Could you check a few things on this drawing? It's one solid part, dimensions in mm from its lowest x, y, z. A direction names the side the tool comes from. Give positions to 0.01 mm unless a question says otherwise; leave off trailing zeros. Loops run counter-clockwise (first coordinate to the right, second up) from the corner with the lowest first, then second, coordinate; pieces in that order, holes last.
Q1. Suppose I cut it at C-C (x = 46). List the corners of the cut face in (y, z) for me, and give its area (3 significant figures).
Q2. I need wall thicknesses on probe 1 along Z at (x, y) = (46, 1.75); probe 2 along Y at (x, z) = (42, 8.25); probe 3 along X at (y, z) = (7.5, 0.5). Which ranges of each line are inside material? Lowest first, please.
Q3. Suppose I cut it at A-A (z = 5). List the corners of the cut face in (x, y) for me, and give its area (3 significant figures).
Q4. For the marked faces 4, 5 and 6, which set-ups out of +Z, -Z, +X, -X, +Y, -Y let a thin tool reach every point of the face, with its end or its side?
Q5. I'm going to push flat-ended pins straight in: P1, Ø6, axis at x = 11, z = 5.5, coming from the +Y side; P2, Ø6, axis at y = 8.5, z = 7.5, coming from the +X side; P3, Ø1.8, axis at y = 9, z = 4.5, coming from the +X side; P4, Ø3, axis at y = 9.5, z = 6.5, coming from the -X side. Where does each tip first touch, or does it pass through?
Q6. Thinking about a two-plate mould opening in X: for the marked faces 1, 2 and 3, which applies, pulls with the +X half, pulls with the -X half, needs draft (parallel to the pull), parting line crosses it, or undercut?
Q7. Suppose I cut it at D-D (z = 1.75). List the corners of the cut face in (x, y) for me.
Q8. Suppose I cut it at B-B (y = 4.25). List the corners of the cut face in (x, z) for me, and give its area (3 significant figures).
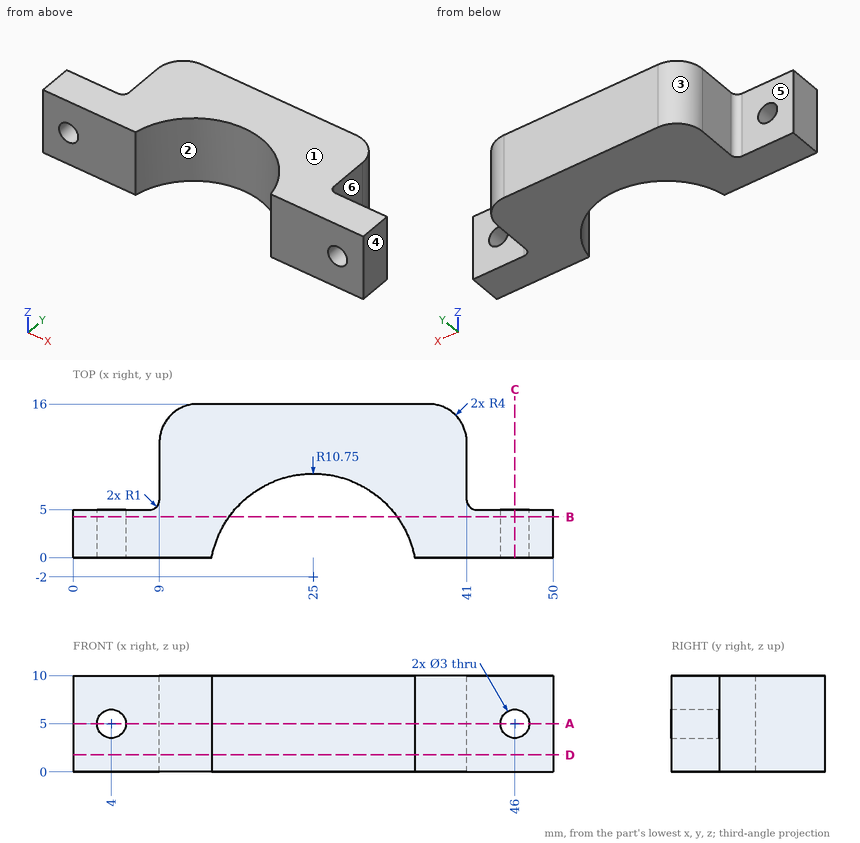
Solutions:
1. outline: (0, 0) - (5, 0) - (5, 3.5) - (0, 3.5) - close; (0, 6.5) - (5, 6.5) - (5, 10) - (0, 10) - close
1. area: 35.0 mm2
2. probe 1: z = 0 to 3.5, 6.5 to 10
2. probe 2: y = 0 to 5
2. probe 3: x = 9 to 19.97, 30.03 to 41
3. outline: (0, 0) - (2.5, 0) - (2.5, 5) - (0, 5) - close; (5.5, 0) - (14.44, 0) arc R10.75 cw to (35.56, 0) - (44.5, 0) - (44.5, 5) - (42, 5) arc R1 cw to (41, 6) - (41, 12) arc R4 ccw to (37, 16) - (13, 16) arc R4 ccw to (9, 12) - (9, 6) arc R1 cw to (8, 5) - (5.5, 5) - close; (47.5, 0) - (50, 0) - (50, 5) - (47.5, 5) - close
3. area: 427 mm2
4. face 4: +Z, -Z, +X, +Y, -Y
4. face 5: +Z, -Z, -X, +Y
4. face 6: +Z, -Z, +X, +Y
5. P1: stops at y = 16
5. P2: stops at x = 41.13
5. P3: stops at x = 41
5. P4: stops at x = 9
6. face 1: needs draft
6. face 2: undercut
6. face 3: pulls with the -X half
7. outline: (0, 0) - (14.44, 0) arc R10.75 cw to (35.56, 0) - (50, 0) - (50, 5) - (42, 5) arc R1 cw to (41, 6) - (41, 12) arc R4 ccw to (37, 16) - (13, 16) arc R4 ccw to (9, 12) - (9, 6) arc R1 cw to (8, 5) - (0, 5) - close
8. outline: (0, 0) - (16.25, 0) - (16.25, 10) - (0, 10) - close; (33.75, 0) - (50, 0) - (50, 10) - (33.75, 10) - close; hole circle Ø3 at (4, 5); hole circle Ø3 at (46, 5)
8. area: 311 mm2
